```python
from build123d import *

# Parameters (mm, degrees)
F2_R     = 5
F3_DEPTH = 65.341817


with BuildPart() as f1:
    # F0 (on Front) → F1 (revolve)
    with BuildSketch(Plane.XZ):
        Polygon((0, 51.4559), (0, 45.307968), (34.767002, 6.023608), (44.309229, 6.023608), (44.309229, 12.047216), (65.340817, 12.047216), (65.340817, 26.136331), (37.162587, 26.136331), (37.162587, 51.4559), align=None)
    revolve(axis=Axis((22.154614, 0, 0), (1, 0, 0)))

    # F2 (on Right) → F3 (cut, through all)
    with BuildSketch(Plane.YZ):
        with Locations((0, 40)):
            Circle(F2_R)
        with Locations((-40, 0)):
            Circle(F2_R)
        with Locations((40, 0)):
            Circle(F2_R)
        with Locations((0, -40)):
            Circle(F2_R)
    extrude(amount=F3_DEPTH, mode=Mode.SUBTRACT)


solid = f1.part
```
Part model, mm, in its own coordinate system. A direction names the side the tool comes from. Coordinates: 2 decimals unless noted, no trailing zeros. Order: outer loops, then holes, each group sorted by start corner. A loop starts at its lowest first (then second) coordinate and runs counter-clockwise, first axis right, second up. Notation, with made-up numbers: (78, 7) - (88, 7) arc R23 cw to (88, 42) - close; hole circle Ø6 at (-8, 86). An arc over 180 degrees is marked (long way). Return JSON: item names as keys, results as strings. Group by question number.
Item 1: Drill centre lines: probe 1 along Z at (x, y) = (41, 0); probe 2 along Y at (x, z) = (37, 0); probe 3 along Y at (x, z) = (12, -2.5). Where is each one in solid material? Low to high. Write a range as from..to.
Item 2: Pin check, flat tips, straight feed: pin 1 (14 mm diameter, centred on y = 0, z = 0, fed in from +X); pin 2 (13 mm diameter, centred on y = 40, z = 0, fed in from +X); pin 3 (5 mm diameter, centred on x = 23.5, y = 31.5, fed in from +Z); pin 4 (19.5 mm diameter, centred on y = 0.5, z = -4.5, fed in from +X). Stop position of each tip, or through.
Item 3: Cut at C-C (x = 61). List the corners of the cut face in (y, z), plus the area to 3 significant figures.
Item 4: Cut at D-D (x = 22.5). List the corners of the cut face in (y, z).
Item 5: Pull direction Y, two halves, no side cores. Call faces 1 (the face through (51.054, 25.515, -5.666)), 2 (the face through (0, 45.5, -0.2)), 3 (the face through (39.605, 2.307, 5.564)): pulls with the +Y half, pulls with the -Y half, needs draft (parallel to the pull), parting line crosses it, or undercut.
Item 6: Cut at A-A (y = 0). List the corners of the cut face in (x, z), plus the area to 3 significant figures.
Item 7: Which spindle directions (+Z, -Z, +X, -X, +Y, -Y) get a long thin tool onto all of the face, cutting with end or side? Do faces 4 (the face through (44.309, -6, -3)), 5 (the face through (22.558, 44.619, -1.915)). Say none if no direction does.
Check values:
{
 "1": {"probe 1": "z = -26.14..-6.02, 6.02..26.14", "probe 2": "y = -51.46..-45, -35..-6.02, 6.02..35, 45..51.46", "probe 3": "y = -51.4..-44.33, -35.67..-31.65, 31.65..35.67, 44.33..51.4"},
 "2": {"pin 1": "stops at x = 44.31", "pin 2": "stops at x = 37.16", "pin 3": "stops at z = 42.51", "pin 4": "stops at x = 65.34"},
 "3": {"outline": "circle Ø52.27 at (0, 0); hole circle Ø24.09 at (0, 0)", "area": "1,690 mm2"},
 "4": {"outline": "circle Ø102.91 at (0, 0); hole circle Ø10 at (-40, 0); hole circle Ø39.77 at (0, 0); hole circle Ø10 at (0, -40); hole circle Ø10 at (0, 40); hole circle Ø10 at (40, 0)"},
 "5": {"face 1": "parting line crosses it", "face 2": "needs draft", "face 3": "undercut"},
 "6": {"outline": "(0, -51.46) - (37.16, -51.46) - (37.16, -45) - (0.27, -45) - (0, -45.31) - close; (0, 45.31) - (0.27, 45) - (37.16, 45) - (37.16, 51.46) - (0, 51.46) - close; (9.12, -35) - (37.16, -35) - (37.16, -26.14) - (65.34, -26.14) - (65.34, -12.05) - (44.31, -12.05) - (44.31, -6.02) - (34.77, -6.02) - close; (9.12, 35) - (34.77, 6.02) - (44.31, 6.02) - (44.31, 12.05) - (65.34, 12.05) - (65.34, 26.14) - (37.16, 26.14) - (37.16, 35) - close", "area": "2,240 mm2"},
 "7": {"face 4": "+X", "face 5": "+X, -X"}
}
